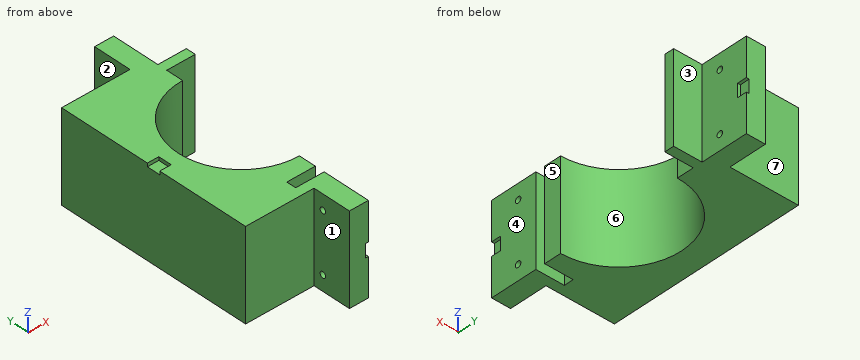
```python
from build123d import *

# Parameters (mm, degrees)
EXTRUDE_1_DEPTH     = 47
SKETCH_2_W          = 47
SKETCH_2_H          = 20
EXTRUDE_2_DEPTH     = 10
SKETCH_5_W          = 47
SKETCH_5_H          = 20
EXTRUDE_5_DEPTH     = 10
SKETCH_6_W          = 15
SKETCH_6_H          = 5
CUT_EXTRUDE_1_DEPTH = 98.514101544
SKETCH_7_W          = 15
SKETCH_7_H          = 5
EXTRUDE_6_DEPTH     = 47
SKETCH_8_W          = 1.5
SKETCH_8_H          = 7
CUT_EXTRUDE_2_DEPTH = 5
SKETCH_10_R         = 1.55
CUT_EXTRUDE_4_DEPTH = 98.514101544
SKETCH_12_R         = 1.55
CUT_EXTRUDE_5_DEPTH = 94.214805691
SKETCH_13_W         = 1.5
SKETCH_13_H         = 7
CUT_EXTRUDE_6_DEPTH = 5
SKETCH_14_W         = 1.8
SKETCH_14_H         = 7
CUT_EXTRUDE_7_DEPTH = 6


with BuildPart() as part:
    # 草图1 → 凸台-拉伸1 (new body)
    with BuildSketch(Plane.XY):
        with BuildLine():
            Line((0, 33), (0, 52))
            Line((0, 52), (-46, 52))
            Line((-46, 52), (-46, -52))
            Line((-46, -52), (0, -52))
            Line((0, -52), (0, -33))
            ThreePointArc((0, -33), (-33, 0), (0, 33))
        make_face()
    extrude(amount=EXTRUDE_1_DEPTH)

    # 草图2 → 凸台-拉伸2 (add)
    with BuildSketch(Plane(origin=(-10, 0, 0), x_dir=(0, 0, -1), z_dir=(1, 0, 0))):
        with Locations((-23.5, 62)):
            Rectangle(SKETCH_2_W, SKETCH_2_H)
    extrude(amount=EXTRUDE_2_DEPTH)

    # 草图5 → 凸台-拉伸5 (add)
    with BuildSketch(Plane(origin=(-10, 0, 0), x_dir=(0, 0, -1), z_dir=(1, 0, 0))):
        with Locations((-23.5, -62)):
            Rectangle(SKETCH_5_W, SKETCH_5_H)
    extrude(amount=EXTRUDE_5_DEPTH)

    # 草图6 → 切除-拉伸1 (cut, through all)
    with BuildSketch(Plane.XY.offset(47)):
        with Locations((-7.5, -44.5)):
            Rectangle(SKETCH_6_W, SKETCH_6_H)
    extrude(amount=-CUT_EXTRUDE_1_DEPTH, mode=Mode.SUBTRACT)

    # 草图7 → 凸台-拉伸6 (add, through all)
    with BuildSketch(Plane.XY.offset(47)):
        with Locations((7.5, 44.5)):
            Rectangle(SKETCH_7_W, SKETCH_7_H)
    extrude(amount=-EXTRUDE_6_DEPTH)

    # 草图8 → 切除-拉伸2 (cut)
    with BuildSketch(Plane.XZ.offset(72)):
        with Locations((-0.75, 23.5)):
            Rectangle(SKETCH_8_W, SKETCH_8_H)
    extrude(amount=-CUT_EXTRUDE_2_DEPTH, mode=Mode.SUBTRACT)

    # 草图10 → 切除-拉伸4 (cut, through all)
    with BuildSketch(Plane(origin=(0, 0, 0), x_dir=(0, 0, -1), z_dir=(1, 0, 0))):
        with Locations((-39, -57)):
            Circle(SKETCH_10_R)
        with Locations((-8, -57)):
            Circle(SKETCH_10_R)
    extrude(amount=-CUT_EXTRUDE_4_DEPTH, mode=Mode.SUBTRACT)

    # 草图12 → 切除-拉伸5 (cut, through all)
    with BuildSketch(Plane.ZY.offset(10)):
        with Locations((8, 57)):
            Circle(SKETCH_12_R)
        with Locations((39, 57)):
            Circle(SKETCH_12_R)
    extrude(amount=-CUT_EXTRUDE_5_DEPTH, mode=Mode.SUBTRACT)

    # 草图13 → 切除-拉伸6 (cut)
    with BuildSketch(Plane(origin=(0, 72, 0), x_dir=(1, 0, 0), z_dir=(0, 1, 0))):
        with Locations((-0.75, -23.5)):
            Rectangle(SKETCH_13_W, SKETCH_13_H)
    extrude(amount=-CUT_EXTRUDE_6_DEPTH, mode=Mode.SUBTRACT)

    # 草图14 → 切除-拉伸7 (cut)
    with BuildSketch(Plane.ZY.offset(46)):
        with Locations((46.1, 0)):
            Rectangle(SKETCH_14_W, SKETCH_14_H)
    extrude(amount=-CUT_EXTRUDE_7_DEPTH, mode=Mode.SUBTRACT)


solid = part.part
```
Could you check a few things on this model? Use its own coordinates, in mm. Face numbers are marked on the shaded views. A direction names the side the tool comes from. Give positions to 0.01 mm unless a question says otherwise; leave off trailing zeros. Loops run counter-clockwise (first coordinate to the right, second up) from the corner with the lowest first, then second, coordinate; pieces in that order, holes last. Notation, with made-up numbers: (35.25, 21.5) - (74.25, 21.5) arc R22 cw to (74.25, 40.5) - close; hole circle Ø8 at (24.25, 78). An arc over 180 degrees is marked (long way). Answer in a Markdown table with one row per item. Add a question column.
Q1. We'd pull the mould along Y, two halves only. Please class the marked faces 5, 6 and 7: +Y half, -Y half, draft (parallel to the pull), parting line (faces both ways), or undercut.
Q2. If we section it at B-B (y = 57): List the corners of the cut face in (x, z) for me, plus the area to 3 significant figures.
Q3. Please list where these lines run through material, in increasing order: L1, parallel to Y at x = -5, z = 8; L2, parallel to Y at x = -4, z = 34; L3, parallel to Y at x = -7.25, z = 8. Write a range as from..to.
Q4. Which directions (+Z, -Z, +X, -X, +Y, -Y) give clear straight access to the entire face, cutting with the end or side of a thin tool? Please do the marked faces 1, 2, 3 and 4.
Q5. If we section it at A-A (z = 39): List the corners of the cut face in (x, y) for me, plus the area to 3 significant figures.
Q6. For pin 1 (20 mm diameter, centred on y = -56.5, z = 35, fed in from +X); pin 2 (1.9 mm diameter, centred on y = 57, z = 39, fed in from +X); pin 3 (2.5 mm diameter, centred on y = 70, z = 23.5, fed in from +X); pin 4 (1 mm diameter, centred on x = -23, z = 25.5, fed in from +Y), each with a flat end and sliding along its axis, tell me the tip position at first contact or that it passes through.
Q7. If we section it at C-C (x = -19): List the corners of the cut face in (y, z) for me, plus the area to 3 significant figures.
Q8. If we section it at D-D (z = 30.5): List the corners of the cut face in (x, y) for me, plus the area to 3 significant figures.
The answers:
| question | item | result |
|---|---|---|
| 1 | face 5 | draft |
| 1 | face 6 | undercut |
| 1 | face 7 | +Y half |
| 2 | outline | (-10, 0) - (0, 0) - (0, 6.45) - (-10, 6.45) - close; (-10, 9.55) - (0, 9.55) - (0, 37.45) - (-10, 37.45) - close; (-10, 40.55) - (0, 40.55) - (0, 47) - (-10, 47) - close |
| 2 | area | 408 mm^2 |
| 3 | L1 | y = -72..-58.55, -55.45..-47, -42..-32.62, 32.62..55.45, 58.55..72 |
| 3 | L2 | y = -72..-47, -42..-32.76, 32.76..72 |
| 3 | L3 | y = -72..-58.55, -55.45..-47, -42..-32.19, 32.19..55.45, 58.55..72 |
| 4 | face 1 | +Z, -Z, -X, -Y |
| 4 | face 2 | +Z, -Z, -X, +Y |
| 4 | face 3 | +Z, -Z, +X, +Y |
| 4 | face 4 | +Z, -Z, +X, -Y |
| 5 | outline | (-46, -52) - (-10, -52) - (-10, -55.45) - (0, -55.45) - (0, -47) - (-15, -47) - (-15, -42) - (0, -42) - (0, -33) arc R33 cw to (0, 33) - (0, 42) - (15, 42) - (15, 47) - (0, 47) - (0, 55.45) - (-10, 55.45) - (-10, 52) - (-46, 52) - close; (-10, -72) - (0, -72) - (0, -58.55) - (-10, -58.55) - close; (-10, 58.55) - (0, 58.55) - (0, 72) - (-10, 72) - close |
| 5 | area | 3,410 mm^2 |
| 6 | pin 1 | stops at x = 0 |
| 6 | pin 2 | passes through |
| 6 | pin 3 | stops at x = -1.5 |
| 6 | pin 4 | stops at y = 52 |
| 7 | outline | (-52, 0) - (-26.98, 0) - (-26.98, 47) - (-52, 47) - close; (26.98, 0) - (52, 0) - (52, 47) - (26.98, 47) - close |
| 7 | area | 2,350 mm^2 |
| 8 | outline | (-46, -52) - (-10, -52) - (-10, -72) - (0, -72) - (0, -47) - (-15, -47) - (-15, -42) - (0, -42) - (0, -33) arc R33 cw to (0, 33) - (0, 42) - (15, 42) - (15, 47) - (0, 47) - (0, 72) - (-10, 72) - (-10, 52) - (-46, 52) - close |
| 8 | area | 3,470 mm^2 |
